Source: three-view drawing plus pictorial views. Frame: mm from the lowest corner of the part. A direction names the side the tool comes from. Round coordinates to 2 decimals unless told otherwise and drop trailing zeros. Loops run counter-clockwise (first coordinate to the right, second up) from the corner with the lowest first, then second, coordinate; pieces in that order, holes last. Notation, with made-up numbers: M 61,-24 L 81,-24 A19 cw 81,4 Z; hole C -17.75,21.25 d6. An arc over 180 degrees is marked long. Answer as a JSON object with one key per item and string values.
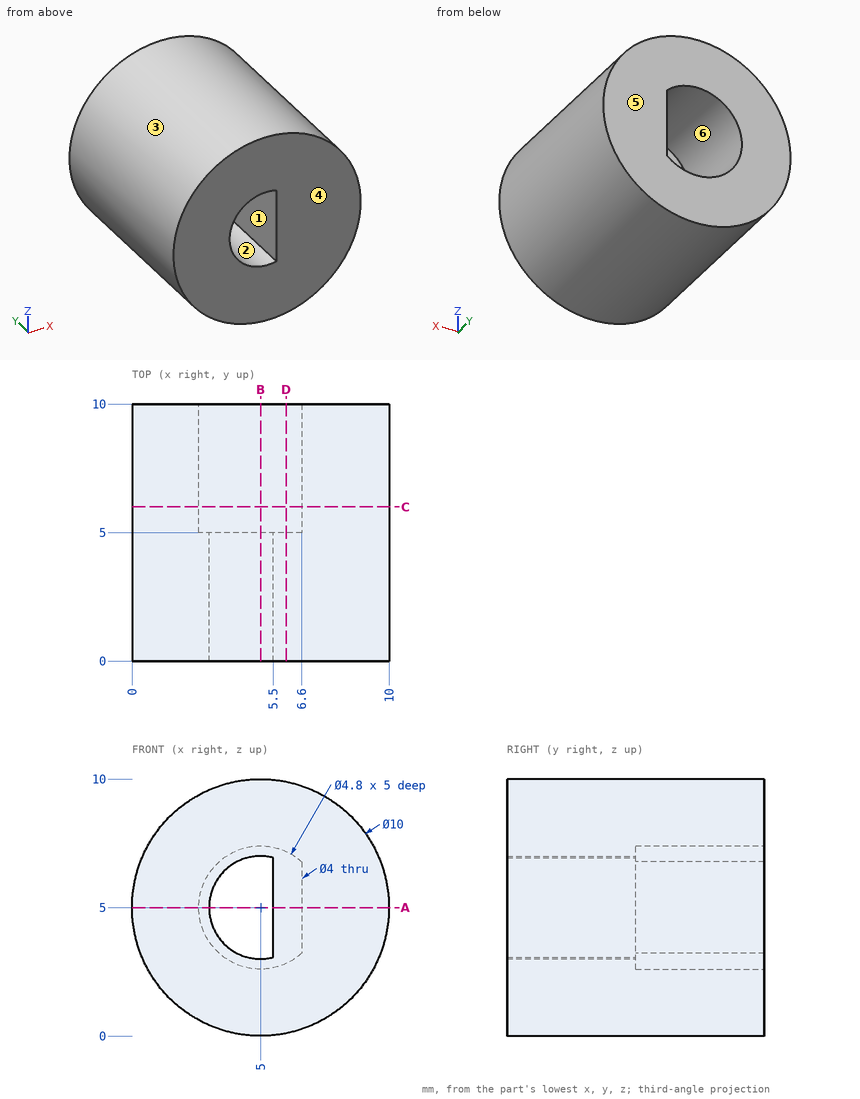
1) Cut plane B-B on x = 5. Return the cut outline in (y, z), and give its area (3 significant figures).
Geometry results:
{"outline": "M 0,0 L 10,0 L 10,2.6 L 5,2.6 L 5,3 L 0,3 Z; M 0,7 L 5,7 L 5,7.4 L 10,7.4 L 10,10 L 0,10 Z", "area": "56.0 mm2"}
2) Cut plane A-A on z = 5. Return the cut outline in (x, y), and give its area (3 significant figures).
Geometry results:
{"outline": "M 0,0 L 3,0 L 3,5 L 2.6,5 L 2.6,10 L 0,10 Z; M 5.5,0 L 10,0 L 10,10 L 6.6,10 L 6.6,5 L 5.5,5 Z", "area": "67.5 mm2"}
3) Cut plane C-C on y = 6. Return the cut outline in (x, z).
Geometry results:
{"outline": "C 5,5 d10; hole M 6.6,3.21 L 6.6,6.79 A2.4 ccw long Z"}
4) Set-up query: the marked faces 5 and 6. Return all of +Z, -Z, +X, -X, +Y, -Y with unobstructed straight access to the full face (end or side cutting, diameter ignored); none if empty.
Geometry results:
{"face 5": "+Z, -Z, +X, -X, +Y", "face 6": "+Y"}
5) Line query: probe 1 along Z at (x, y) = (5, 2.9); probe 2 along Z at (x, y) = (5, 6.5); probe 3 along X at (y, z) = (7, 3.5). Output: solid intervals per line, ascending.
Geometry results:
{"probe 1": "0 to 3, 7 to 10", "probe 2": "0 to 2.6, 7.4 to 10", "probe 3": "0.23 to 3.13, 6.6 to 9.77"}
6) Pull-direction query (Z, two-part tool) for the marked faces 1, 2, 3 and 4; classes: +Z half, -Z half, draft (parallel to the pull), parting line (faces both ways), or undercut.
Geometry results:
{"face 1": "undercut", "face 2": "undercut", "face 3": "parting line", "face 4": "draft"}
7) First-contact query: pin 1 (2.5 mm diameter, centred on x = 5, z = 5, fed in from +Y); pin 2 (2 mm diameter, centred on y = 8, z = 1.5, fed in from -X); pin 3 (1 mm diameter, centred on x = 1.5, y = 3, fed in from +Z). Flat tips, straight axial feed; report the tip coordinate or a pass-through.
Geometry results:
{"pin 1": "y = 5", "pin 2": "x = 0.67", "pin 3": "z = 9"}
8) Cut plane D-D on x = 6. Return the cut outline in (y, z).
Geometry results:
{"outline": "M 0,0.1 L 10,0.1 L 10,2.82 L 5,2.82 L 5,7.18 L 10,7.18 L 10,9.9 L 0,9.9 Z"}
